Part model, mm, in its own coordinate system. A direction names the side the tool comes from. Give positions to 0.01 mm unless a question says otherwise; leave off trailing zeros. Write each loop counter-clockwise with the first axis right and the second up, starting at its lowest first coordinate (ties: lowest second). Pieces come first, ordered by that corner, then holes. Notation, with made-up numbers: (-34, -30) - (6, -30) arc R26 cw to (6, -16) - close; hole circle Ø3 at (18, 45.25). An arc over 180 degrees is marked (long way). Answer in a Markdown table with one row per item. Add a question column.
1. Pull direction Y, two halves, no side cores. Call faces 1 (the flat face through (16, 57, 5)), 2 (the cylindrical face through (13.5, 6.57, 2.46)), 3 (the flat face through (13, 0, 2)): released by +Y, released by -Y, zero draft, split by the parting line, or undercut.
2. Drop flat-ended pins along their axis: pin 1 Ø2 at (x, z) = (18.5, 2.5) entering from +Y; pin 2 Ø1 at (x, z) = (3, 3) entering from +Y; pin 3 Ø1 at (y, z) = (16, 3.5) entering from +X; pin 4 Ø2.5 at (x, y) = (5, 54.5) entering from -Z. Give the stop position or say it passes through.
3. Probe line 1 along Y through (x, z) = (10, 3.7); line 2 along Y through (x, z) = (16, 0.95); line 3 along Y through (x, z) = (19.5, 4.1). List the from-to ranges inside material, lowest first.
4. Band-saw the part on D-D on y = 64. Write the cut outline in (x, z).
5. Band-saw the part on C-C on y = 6.5. Write the cut outline in (x, z).
6. Which spindle directions (+Z, -Z, +X, -X, +Y, -Y) get a long thin tool onto all of the face, cutting with end or side? Do faces 4 (the flat face through (4.496, 74.528, 2.465)), 5 (the flat face through (15, 76.5, 2)), 6 (the flat face through (19.614, 82.911, 2.465)). Say none if no direction does.
7. Band-saw the part on B-B on z = 3.3. Write the cut outline in (x, y).
8. Band-saw the part on A-A on x = 10. Write the cut outline in (y, z), plus the area to 3 significant figures.
```python
from build123d import *

# Parameters (mm, degrees)
ESQUISSE1_R        = 1.5
ESQUISSE1_W        = 5
ESQUISSE1_H        = 18
BOSS_EXTRU_1_DEPTH = 5
CONG_3_R           = 1.5


with BuildPart() as part:
    # Esquisse1 → Boss.-Extru.1 (new body)
    with BuildSketch(Plane.XY):
        with BuildLine():
            Line((0, 10), (0, 0))
            Line((0, 0), (26.554131445, 0))
            Line((26.554131445, 0), (24.226405413, 76.5))
            Line((24.226405413, 76.5), (14.870448313, 89.504102342))
            ThreePointArc((14.870448313, 89.504102342), (8.034842814, 91.669052587), (4.005728082, 85.7378852))
            Line((4.005728082, 85.7378852), (5, 63))
            Line((5, 63), (0, 63))
            Line((0, 63), (0, 51))
            Line((0, 51), (11, 51))
            Line((11, 51), (20, 51))
            Line((20, 51), (20, 10))
            Line((20, 10), (11, 10))
            Line((11, 10), (0, 10))
        make_face()
        with Locations((5, 54.5)):
            Circle(ESQUISSE1_R, mode=Mode.SUBTRACT)
        with Locations((15, 6.5)):
            Circle(ESQUISSE1_R, mode=Mode.SUBTRACT)
        with Locations((5, 6.5)):
            Circle(ESQUISSE1_R, mode=Mode.SUBTRACT)
        with Locations((10, 86)):
            Circle(ESQUISSE1_R, mode=Mode.SUBTRACT)
        with Locations((15.02885683, 67.5)):
            Rectangle(ESQUISSE1_W, ESQUISSE1_H, mode=Mode.SUBTRACT)
    extrude(amount=BOSS_EXTRU_1_DEPTH)

    # Congé3
    cong_3_edges = [part.edges().sort_by_distance(p)[0] for p in [
        (0, 63, 2.5),
    ]]
    fillet(cong_3_edges, radius=CONG_3_R)


solid = part.part
```
Values:
| question | item | result |
|---|---|---|
| 1 | face 1 | zero draft |
| 1 | face 2 | undercut |
| 1 | face 3 | released by -Y |
| 2 | pin 1 | stops at y = 85.85 |
| 2 | pin 2 | stops at y = 63 |
| 2 | pin 3 | stops at x = 26.08 |
| 2 | pin 4 | passes through |
| 3 | line 1 | y = 0 to 10, 51 to 84.5, 87.5 to 92 |
| 3 | line 2 | y = 0 to 5.38, 7.62 to 10, 51 to 58.5, 76.5 to 87.93 |
| 3 | line 3 | y = 0 to 10, 51 to 83.07 |
| 4 | outline | (4.96, 0) - (12.53, 0) - (12.53, 5) - (4.96, 5) - close; (17.53, 0) - (24.61, 0) - (24.61, 5) - (17.53, 5) - close |
| 5 | outline | (0, 0) - (3.5, 0) - (3.5, 5) - (0, 5) - close; (6.5, 0) - (13.5, 0) - (13.5, 5) - (6.5, 5) - close; (16.5, 0) - (26.36, 0) - (26.36, 5) - (16.5, 5) - close |
| 6 | face 4 | +Z, -Z, -X |
| 6 | face 5 | +Z, -Z |
| 6 | face 6 | +Z, -Z, +X, +Y |
| 7 | outline | (0, 0) - (26.55, 0) - (24.23, 76.5) - (14.87, 89.5) arc R6 ccw to (4.01, 85.74) - (5, 63) - (1.5, 63) arc R1.5 ccw to (0, 61.5) - (0, 51) - (20, 51) - (20, 10) - (0, 10) - close; hole circle Ø3 at (5, 6.5); hole circle Ø3 at (5, 54.5); hole circle Ø3 at (10, 86); hole (12.53, 58.5) - (17.53, 58.5) - (17.53, 76.5) - (12.53, 76.5) - close; hole circle Ø3 at (15, 6.5) |
| 8 | outline | (0, 0) - (10, 0) - (10, 5) - (0, 5) - close; (51, 0) - (84.5, 0) - (84.5, 5) - (51, 5) - close; (87.5, 0) - (92, 0) - (92, 5) - (87.5, 5) - close |
| 8 | area | 240 mm² |
